Read the model definition and answer for the solid it produces. Units are mm, in the model's axes. A direction names the side the tool comes from. Round coordinates to 2 decimals unless told otherwise and drop trailing zeros. Write each loop counter-clockwise with the first axis right and the second up, starting at its lowest first coordinate (ties: lowest second). Pieces come first, ordered by that corner, then holes. Notation, with made-up numbers: (72, 89) - (126, 89) arc R28 ccw to (126, 117) - close; hole circle Ø3 at (3.25, 86.25). An arc over 180 degrees is marked (long way). Use one line per item in the form item = value. Start each with the question number.
1) The part is cut by section A-A, the plane y = 0.8. Give the vertices of the cut face in (x, z), plus the area to 3 significant figures.
2) The part is cut by section C-C, the plane y = -0.45. Give the vertices of the cut face in (x, z), plus the area to 3 significant figures.
3) Consider line 1 along X through (y, z) = (0.1, 1); line 2 along Y through (x, z) = (5.5, 2); line 3 along X through (y, z) = (-0.05, -4). Determine where each line is inside the solid, lowest interval first. Write a range as from..to.
4) Each of these flat-tipped pins is pushed along its axis until it touches: pin 1 (5 mm diameter, centred on x = -2, z = -4.5, fed in from -Y); pin 2 (0.5 mm diameter, centred on x = 7, y = 0.5, fed in from +Z); pin 3 (0.8 mm diameter, centred on x = -7, y = 0.5, fed in from -Z). Where does it stop, or does it pass through?
5) For a pull along X with two mould halves and no side action, classify faces 6 (the face through (7, 1.2, 0.7)), 7 (the face through (6.5, 1, 1)), 8 (the face through (7.5, 0, 1)), 9 (the face through (-4.619, -0.394, 5.163)) as released by +X, released by -X, zero draft, split by the parting line, or undercut.
6) For faces 1 (the face through (3.2, -0.8, -4.2)), 2 (the face through (-7, 0.5, -1.5)), 3 (the face through (0, -1.8, 0)), 4 (the face through (-6.5, 1, 1)), 5 (the face through (7, 1, 2.923)), determine the directions among +Z, -Z, +X, -X, +Y, -Y from which every point of the face is accessible in a straight line to the end or side of a thin tool.
from build123d import *

# Parameters (mm, degrees)
F1_DEPTH = 0.8
F2_R     = 5
F3_R     = 1
F4_R     = 5
F5_DEPTH = 1
F6_SIZE2 = 2.99999
F6_SIZE  = 0.99999
F8_DEPTH = 1


# Not quite as in the source:
# - a fillet or chamfer is up to 0.001 mm smaller than in the source, because OpenCascade refuses the exact size


with BuildPart() as f1:
    # F0 (on Front) → F1 (new body)
    with BuildSketch(Plane.XZ):
        Polygon((7.5, 3.5), (2.3038475773, 6.5), (-2.3038475773, 6.5), (-7.5, 3.5), (-7.5, -6.5), (7.5, -6.5), align=None)
    extrude(amount=F1_DEPTH)

    # F2
    f2_edges = [f1.edges().sort_by_distance(p)[0] for p in [
        (7.5, -0.4, -6.5),
        (-7.5, -0.4, -6.5),
    ]]
    fillet(f2_edges, radius=F2_R)

    # F3
    f3_edges = [f1.edges().sort_by_distance(p)[0] for p in [
        (7.5, -0.4, 3.5),
        (-7.5, -0.4, 3.5),
    ]]
    fillet(f3_edges, radius=F3_R)

    # F4 (on face) → F5 (join)
    with BuildSketch(Plane.XZ.offset(0.8)):
        Circle(F4_R)
    extrude(amount=F5_DEPTH)

    # F6 (size 1 and 3 in the source; OpenCascade refuses exactly that, so slightly less here)
    f6_edges = [f1.edges().sort_by_distance(p)[0] for p in [
        (-5, -1.8, 0),
    ]]
    f6_side = f1.faces().sort_by_distance((-5, -1.3, 0))[0]
    chamfer(f6_edges, length=F6_SIZE, length2=F6_SIZE2, reference=f6_side)

    # F7 (on face) → F8 (join)
    with BuildSketch(Plane.YZ.offset(7.5)):
        Polygon((1.4, 2.9226497308), (0, 2.9226497308), (0, -1.5), (1, -1.5), align=None)
    extrude(amount=-F8_DEPTH)

    # F9: F1 across plane


with BuildPart() as f1_1:
    add(f1.part)
    add(f1.part.mirror(Plane.YZ))


solid = f1_1.part
Geometry results:
q1.outline = (-7.5, -1.5) - (-6.5, -1.5) - (-6.5, 2.92) - (-7.5, 2.92) - close; (6.5, -1.5) - (7.5, -1.5) - (7.5, 2.92) - (6.5, 2.92) - close
q1.area = 8.85 mm2
q2.outline = (-7.5, -1.5) arc R5 ccw to (-2.5, -6.5) - (2.5, -6.5) arc R5 ccw to (7.5, -1.5) - (7.5, 2.92) arc R1 ccw to (7, 3.79) - (2.3, 6.5) - (-2.3, 6.5) - (-7, 3.79) arc R1 ccw to (-7.5, 2.92) - close
q2.area = 169 mm2
q3.line_1 = -7.5..-6.5, 6.5..7.5
q3.line_2 = -0.8..0
q3.line_3 = -6.83..6.83
q4.pin_1 = -1.66
q4.pin_2 = 2.92
q4.pin_3 = -1.5
q5.face_6 = zero draft
q5.face_7 = undercut
q5.face_8 = released by +X
q5.face_9 = released by -X
q6.face_1 = -Y
q6.face_2 = -Z, +X, -X, +Y
q6.face_3 = +Z, -Z, +X, -X, -Y
q6.face_4 = +Z, -Z, +Y
q6.face_5 = +Z, +X, -X, +Y
